Autodesk Fusion 360 part; units mm, degrees
sketch "Sketch1" plane through (0, 0, 0) normal (1, 0, 0) x (0, 0, -1)
  circle A0 centre (0, 0) radius 21.5
  line L0 (19.85, -10.1) -> (-19.85, -10.1)
  line L1 (-19.85, -10.1) -> (-19.85, 10.1)
  line L2 (-19.85, 10.1) -> (19.85, 10.1)
  line L3 (19.85, 10.1) -> (19.85, -10.1)
  line L4 (19.85, -10.1) -> (-19.85, 10.1) construction
  line L5 (-19.85, -10.1) -> (19.85, 10.1) construction
  circle A1 centre (0, 0) radius 24
  line L6 (10.25, -26.5) -> (-10.25, -26.5)
  line L7 (-10.25, -26.5) -> (-10.25, 26.5)
  line L8 (-10.25, 26.5) -> (10.25, 26.5)
  line L9 (10.25, 26.5) -> (10.25, -26.5)
  line L10 (10.25, -26.5) -> (-10.25, 26.5) construction
  line L11 (-10.25, -26.5) -> (10.25, 26.5) construction
  line L12 (-10.25, 16.5) -> (10.25, 16.5)
  line L13 (-10.25, -16.5) -> (10.25, -16.5)
  dimension "CaseInnerDiameter" = 43
  dimension "BatteryLength" = 39.7
  dimension "BatteryWidth" = 20.2
  dimension "CaseWallThickness" = 2.5
  dimension "LugWidth" = 20.5
  dimension "StrapCutout" = 53
  dimension "UpperLugInset" = 10
  dimension "LowerLugInset" = 10
sketch "Sketch19" plane through (0, 0, 0) normal (0, 1, 0) x (1, 0, 0)
  circle A0 centre (-0.2453, 29.9832) radius 1.725
  circle A1 centre (0.3438, 29.9967) radius 2.35
  dimension "d142" = 3.45
  dimension "d145" = 4.7
extrude "Extrude28" add sketch "Sketch19" against normal blind 1 contours A0 | A1 makes body 1
extrude "Extrude27" add sketch "Sketch19" along normal blind 6 separate body contours A0 makes body 2
combine "Combine3" operation add target body 1 tool bodies 2
chamfer "Chamfer9" distance 0.5 angle 45 1 edges at (-1.8536, 6, -29.3595) on bodies 1
equation "StrapCutout = CaseInnerDiameter + 10 mm"
equation "BottomCaseLipChamfer = 1.20 mm"
equation "UpperCaseThickness = 5.77 mm"
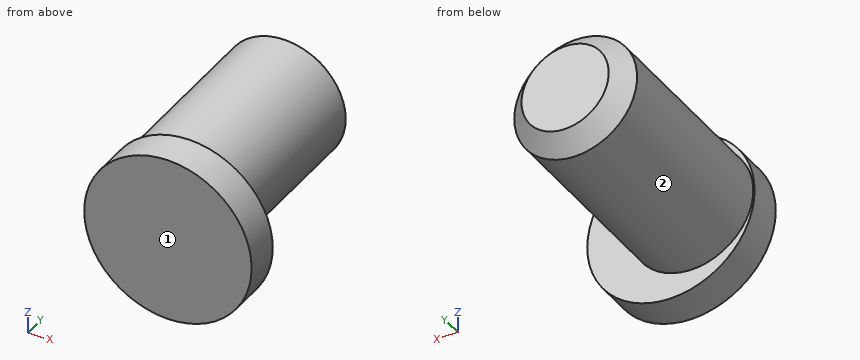
Input: part model. Units: mm. Frame: model coordinates. Face numbers are marked on the shaded views. A direction names the side the tool comes from. Give positions to 0.01 mm unless a question says otherwise; leave off trailing zeros. Write each loop counter-clockwise with the first axis right and the second up, starting at its lowest first coordinate (ties: lowest second). Pieces come first, ordered by that corner, then holes. Notation, with made-up numbers: M -29,-32 L -15,-32 A36 cw -15,3 Z; hole C 39.25,74.25 d4. An arc over 180 degrees is marked long. Use one line per item in the form item = value.
1. Reachability of the marked faces 1 and 2 from +Z, -Z, +X, -X, +Y, -Y: full face, straight path, thin tool, end or side. Return the list, or none.
Outcome:
face_1 = +Z, -Z, +X, -X, -Y
face_2 = +Y
2. First-contact query: P1, Ø1, axis at x = 1, y = 0, coming from the -Z side; P2, Ø1.5, axis at x = 1, y = 2, coming from the -Z side; P3, Ø2, axis at y = 0.5, z = -28.5, coming from the -X side. Flat tips, straight axial feed; report the tip coordinate or a pass-through.
Outcome:
P1 = -32.34
P2 = -31.64
P3 = -1.92
3. Cut plane A-A on z = -28.15. Return loops of the section in (x, y), and give its area (3 significant figures).
Outcome:
outline = M -1.11,-1 L 1.8,-1 L 1.8,0 L -1.11,0 Z
area = 2.91 mm²
4. Cut plane B-B on y = 0.5. Return loops of the section in (x, z) (3 decimals).
Outcome:
outline = C -0.245,-29.983 d3.45
5. Cut plane C-C on y = 5.75. Return loops of the section in (x, z) (3 decimals), and give its area (3 significant figures).
Outcome:
outline = C -0.245,-29.983 d2.95
area = 6.83 mm²
6. Ray query, L1, parallel to Y at x = 2.4, z = -29.2; L2, parallel to Z at x = -0.15, y = 2.25; L3, parallel to X at y = 4.5, z = -31.2. Return the intervals inside material, ascending.
Outcome:
L1 = -1 to 0
L2 = -31.71 to -28.26
L3 = -1.47 to 0.98
